Autodesk Inventor part; units mm, degrees
ref_plane "YZ Plane" through (0, 0, 0) normal (1, 0, 0) x (0, 1, 0)
ref_plane "XZ Plane" through (0, 0, 0) normal (0, 1, 0) x (-1, 0, 0)
ref_plane "XY Plane" through (0, 0, 0) normal (0, 0, 1) x (1, 0, 0)
sketch "Sketch1" plane through (0, 0, 0) normal (0, 1, 0) x (-1, 0, 0)
  circle A0 centre (0, 0) radius 87.5
  dimension "d0" = 175
extrude "Plate1" add sketch "Sketch1" along normal blind 3
sketch "Sketch2" plane through (0, 3, 0) normal (0, 1, 0) x (1, 0, 0)
  line L0 (-40, -40) -> (40, -40) construction
  line L1 (40, -40) -> (40, 40) construction
  line L2 (40, 40) -> (-40, 40) construction
  line L3 (-40, 40) -> (-40, -40) construction
  line L4 (40, -40) -> (-40, 40) construction
  circle A0 centre (0, 0) radius 87.5
  line L5 (0, 0) -> (0, -87.5) construction
  circle A1 centre (0, -74) radius 6
  dimension "d2" = 80
  dimension "d3" = 80
  dimension "d16" = 12
  dimension "d17" = 13.5
extrude "Extrusion1" cut sketch "Sketch2" against normal through all contours A1
pattern_circular "Circular Pattern1" count 4 over 360 about axis through (0, -10, 0) along (0, 1, 0) of "Extrusion1"
equation "\"d1\" = Thickness"
equation "\"BendReliefWidth\" = Thickness"
equation "\"BendReliefDepth\" = 0.5 * Thickness"
equation "\"CornerReliefSize\" = 4 * Thickness"
equation "\"MinimumRemnant\" = 2 * Thickness"
equation "\"TransitionRadius\" = BendRadius"
equation "\"JacobiRadiusSize\" = BendRadius"
equation "\"GapSize\" = Thickness"
properties part number "MSC 126 flange base tube" material "Stainless Steel"
Source: CAD feature listing. Evaluate the final solid. Frame: model axes, mm. Give positions to 0.01 mm unless a question says otherwise; leave off trailing zeros. Write each loop counter-clockwise with the first axis right and the second up, starting at its lowest first coordinate (ties: lowest second). Pieces come first, ordered by that corner, then holes. Notation, with made-up numbers: M 77.5,33.5 L 118.5,33.5 A27 ccw 118.5,67.5 Z; hole C 70,5.25 d11. An arc over 180 degrees is marked long. Return JSON: item names as keys, results as strings. Group by question number.
1) Pull-direction query (Z, two-part tool) for faces 1 (the face through (64.49, 1.48, -59.14)), 2 (the face through (0.78, 1.52, -68.05)), 3 (the face through (68.05, 1.52, 0.78)), 4 (the face through (1, 3, 1)); classes: pulls with the +Z half, pulls with the -Z half, needs draft (parallel to the pull), parting line crosses it, or undercut.
2) Cut plane D-D, the plane z = 74. Output: boundary loops of the cut face in (x, y).
3) Pin query (flat end, axial travel): P1, Ø9.5, axis at x = 74, z = 0, coming from the +Y side; P2, Ø1.5, axis at x = 68, y = 2, coming from the -Z side. Return the tip coordinate at first contact, or that it passes through.
4) Material intervals for line 1 along Z through (x, y) = (0, 0.8); line 2 along Z through (x, y) = (2, 0.2); line 3 along X through (y, z) = (1.1, 74), sorted ascending. Write a range as [from, to].
5) Cut plane A-A, the plane x = 0. Output: boundary loops of the cut face in (y, z), plus the area to 3 significant figures.
6) Cut plane C-C, the plane y = 2.55. Output: boundary loops of the cut face in (x, z), plus the area to 3 significant figures.
7) Cut plane B-B, the plane z = -3.5. Output: boundary loops of the cut face in (x, y), plus the area to 3 significant figures.
Recorded:
{
 "1": {"face 1": "parting line crosses it", "face 2": "undercut", "face 3": "undercut", "face 4": "needs draft"},
 "2": {"outline": "M -46.69,0 L -6,0 L -6,3 L -46.69,3 Z; M 6,0 L 46.69,0 L 46.69,3 L 6,3 Z"},
 "3": {"P1": "passes through", "P2": "stops at z = -55.98"},
 "4": {"line 1": "z = [-87.5, -80], [-68, 68], [80, 87.5]", "line 2": "z = [-87.48, -79.66], [-68.34, 68.34], [79.66, 87.48]", "line 3": "x = [-46.69, -6], [6, 46.69]"},
 "5": {"outline": "M 0,-87.5 L 3,-87.5 L 3,-80 L 0,-80 Z; M 0,-68 L 3,-68 L 3,68 L 0,68 Z; M 0,80 L 3,80 L 3,87.5 L 0,87.5 Z", "area": "453 mm²"},
 "6": {"outline": "C 0,0 d175; hole C -74,0 d12; hole C 0,-74 d12; hole C 0,74 d12; hole C 74,0 d12", "area": "23,600 mm²"},
 "7": {"outline": "M -87.43,0 L -78.87,0 L -78.87,3 L -87.43,3 Z; M -69.13,0 L 69.13,0 L 69.13,3 L -69.13,3 Z; M 78.87,0 L 87.43,0 L 87.43,3 L 78.87,3 Z", "area": "466 mm²"}
}
